Part model, mm, in its own coordinate system. A direction names the side the tool comes from. Round coordinates to 2 decimals unless told otherwise and drop trailing zeros. Write each loop counter-clockwise with the first axis right and the second up, starting at its lowest first coordinate (ties: lowest second). Pieces come first, ordered by that corner, then holes.
```python
from build123d import *

# Parameters (mm, degrees)
F1_DEPTH = 50.8
F2_R     = 5
F3_DEPTH = 6.351
F5_D     = 4.776


with BuildPart() as f1:
    # F0 (on Front) → F1 (new body)
    with BuildSketch(Plane.XZ):
        Polygon((0, 50.8), (0, 0), (50.8, 0), (50.8, 6.35), (6.35, 6.35), (6.35, 50.8), align=None)
    extrude(amount=F1_DEPTH)

    # F2 (on face) → F3 (cut, through all)
    with BuildSketch(Plane.YZ.offset(6.35)):
        with Locations((-25.4, 38.738448)):
            Circle(F2_R)
    extrude(amount=-F3_DEPTH, mode=Mode.SUBTRACT)

    # F5 (through all)
    with Locations(Plane.YZ.offset(6.35)):
        with Locations((-25.4, 28.738448)):
            Hole(F5_D / 2)


solid = f1.part
```
Q1. Cut at B-B on z = 40. Write the cut outline in (x, y).
Values follow:
outline: (0, -50.8) - (6.35, -50.8) - (6.35, -30.24) - (0, -30.24) - close; (0, -20.56) - (6.35, -20.56) - (6.35, 0) - (0, 0) - close
Q2. Cut at A-A on y = -25.4. Write the cut outline in (x, z), plus the area to 3 significant figures.
Values follow:
outline: (0, 0) - (50.8, 0) - (50.8, 6.35) - (6.35, 6.35) - (6.35, 26.35) - (0, 26.35) - close; (0, 31.13) - (6.35, 31.13) - (6.35, 33.74) - (0, 33.74) - close; (0, 43.74) - (6.35, 43.74) - (6.35, 50.8) - (0, 50.8) - close
area: 511 mm2
Q3. Wall check: L1, parallel to Z at x = 1.5, y = -25.4; L2, parallel to Z at x = 1, y = -25; L3, parallel to X at y = -3, z = 38.5. Give the ranges that are in metal, low to high.
Values follow:
L1: z = 0 to 26.35, 31.13 to 33.74, 43.74 to 50.8
L2: z = 0 to 26.38, 31.09 to 33.75, 43.72 to 50.8
L3: x = 0 to 6.35
Q4. Cut at D-D on z = 23. Write the cut outline in (x, y).
Values follow:
outline: (0, -50.8) - (6.35, -50.8) - (6.35, 0) - (0, 0) - close
Q5. Cut at C-C on y = -40. Write the cut outline in (x, z).
Values follow:
outline: (0, 0) - (50.8, 0) - (50.8, 6.35) - (6.35, 6.35) - (6.35, 50.8) - (0, 50.8) - close
Q6. Drop flat-ended pins along their axis: pin 1 (8 mm diameter, centred on y = -45, z = 21, fed in from +X); pin 2 (1 mm diameter, centred on x = 37, y = -17.5, fed in from +Z); pin 3 (4 mm diameter, centred on y = -25.4, z = 28.74, fed in from -X). Give the stop position or say it passes through.
Values follow:
pin 1: stops at x = 6.35
pin 2: stops at z = 6.35
pin 3: passes through
Q7. Mould opens along Z. For faces 1 (the cylindrical face through (3.131, -27.678, 29.456)), 2 (the flat face through (3, -25, 50.8)), 3 (the flat face through (14, 0, 5)) say: +Z half, -Z half, draft (parallel to the pull), parting line (faces both ways), or undercut.
Values follow:
face 1: undercut
face 2: +Z half
face 3: draft
Q8. Which spindle directions (+Z, -Z, +X, -X, +Y, -Y) get a long thin tool onto all of the face, cutting with end or side? Do faces 4 (the flat face through (6.35, -25, 23)), 5 (the flat face through (25, -25, 0)). Say none if no direction does.
Values follow:
face 4: +Z, +X, +Y, -Y
face 5: -Z, +X, -X, +Y, -Y
